Answer from the drawing. Dimensions are ordinates in mm from the lowest x, y and z of the part. A direction names the side the tool comes from. Round coordinates to 2 decimals unless told otherwise and drop trailing zeros. Order: outer loops, then holes, each group sorted by start corner. A loop starts at its lowest first (then second) coordinate and runs counter-clockwise, first axis right, second up. Notation, with made-up numbers: (64, 86.25) -> (70, 86.25) arc R27 ccw to (70, 116.25) -> close; hole circle Ø3 at (85, 16). An arc over 180 degrees is marked (long way). Use a Markdown table: item, result. Add a question column.
Item 1: A cutting plane is placed at A-A, the plane y = 7.35. Determine the outline of the cut face in (x, z).
Item 2: A tool of negligible diameter and unlimited length cuts with its end or side. For the marked faces 5, 6, 7, 8 and 9, from which of +Z, -Z, +X, -X, +Y, -Y can it reach the whole face along a straight path? Write none if from no direction.
Item 3: Find the intervals of material crossed by L1, parallel to Z at x = 3.75, y = 8.25; L2, parallel to Y at x = 7, z = 2.3; L3, parallel to Z at x = 3.25, y = 11, in increasing order. Write a range as [from, to].
Item 4: A cutting plane is placed at B-B, the plane z = 32.45. Determine the outline of the cut face in (x, y).
Item 5: A cutting plane is placed at C-C, the plane y = 17. Determine the outline of the cut face in (x, z) (1 decimal).
Item 6: A cutting plane is placed at D-D, the plane z = 6.5. Determine the outline of the cut face in (x, y) (1 decimal), plus the area to 3 significant figures.
Item 7: Flat-ended cylindrical pins translate along their axes: P1, Ø3, axis at y = 6.5, z = 5, coming from the +X side; P2, Ø2, axis at y = 16.5, z = 33.5, coming from the +X side; P3, Ø1.2, axis at y = 7, z = 5.5, coming from the -X side; P4, Ø4, axis at x = 7.5, y = 9, coming from the -Z side. Find the tip coordinate at first contact, or state that the pin passes through.
Item 8: For a pull along X with two mould halves and no side action, classify the marked faces 1, 2, 3 and 4 as +X half, -X half, draft (parallel to the pull), parting line (faces both ways), or undercut.
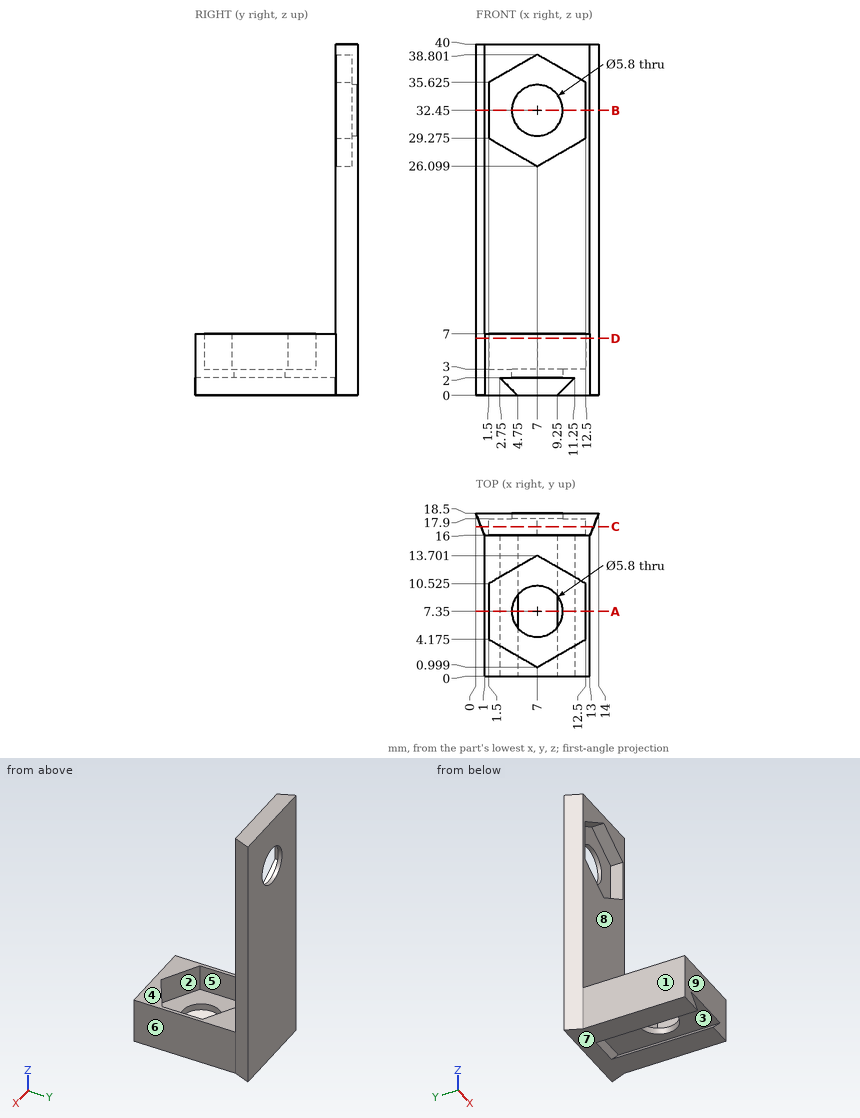
Reported:
| question | item | result |
|---|---|---|
| 1 | outline | (1, 0) -> (4.75, 0) -> (2.75, 2) -> (4.1, 2) -> (4.1, 3) -> (1.5, 3) -> (1.5, 7) -> (1, 7) -> close; (9.25, 0) -> (13, 0) -> (13, 7) -> (12.5, 7) -> (12.5, 3) -> (9.9, 3) -> (9.9, 2) -> (11.25, 2) -> close |
| 2 | face 5 | +Z |
| 2 | face 6 | +Z, -Z, +X, -Y |
| 2 | face 7 | -Z, +X, -X, +Y, -Y |
| 2 | face 8 | +Z, +X, -X, -Y |
| 2 | face 9 | +Z, -Z, +X, -X, -Y |
| 3 | L1 | [0, 1], [2, 3] |
| 3 | L2 | [0, 4.45], [10.25, 18.5] |
| 3 | L3 | [0, 1.5], [2, 3] |
| 4 | outline | (0, 18.5) -> (1, 16) -> (1.5, 16) -> (1.5, 17.9) -> (4.1, 17.9) -> (4.1, 18.5) -> close; (9.9, 17.9) -> (12.5, 17.9) -> (12.5, 16) -> (13, 16) -> (14, 18.5) -> (9.9, 18.5) -> close |
| 5 | outline | (0.6, 0) -> (13.4, 0) -> (13.4, 40) -> (0.6, 40) -> close; hole (1.5, 29.3) -> (7, 26.1) -> (12.5, 29.3) -> (12.5, 35.6) -> (7, 38.8) -> (1.5, 35.6) -> close |
| 6 | outline | (0, 18.5) -> (1, 16) -> (1, 0) -> (13, 0) -> (13, 16) -> (14, 18.5) -> close; hole (1.5, 4.2) -> (7, 1) -> (12.5, 4.2) -> (12.5, 10.5) -> (7, 13.7) -> (1.5, 10.5) -> close |
| 6 | area | 120 mm² |
| 7 | P1 | x = 13 |
| 7 | P2 | x = 13.6 |
| 7 | P3 | x = 1 |
| 7 | P4 | z = 0 |
| 8 | face 1 | -X half |
| 8 | face 2 | undercut |
| 8 | face 3 | undercut |
| 8 | face 4 | draft |
